Read the model definition and answer for the solid it produces. Units are mm, in the model's axes. Face numbers are marked on the shaded views. A direction names the side the tool comes from. Coordinates: 2 decimals unless noted, no trailing zeros. Order: outer loops, then holes, each group sorted by start corner. A loop starts at its lowest first (then second) coordinate and runs counter-clockwise, first axis right, second up. Notation, with made-up numbers: M 88.5,-19 L 113.5,-19 A11 ccw 113.5,-6 Z; hole C 19,77.25 d6. An arc over 180 degrees is marked long. One line per question, with ' | ' between items. Start each with the question number.
1) A tool of negligible diameter and unlimited length cuts with its end or side. For the marked faces 4, 5, 6 and 7, from which of +Z, -Z, +X, -X, +Y, -Y can it reach the whole face along a straight path? Write none if from no direction.
2) Find section A-A, the plane z = 13.2. Write down the section's boundary in (x, y).
3) Given P1, Ø4, axis at x = -12, z = 6, coming from the -Y side; P2, Ø2, axis at x = 2.5, z = -4.5, coming from the +Y side; P3, Ø2.5, axis at x = -8.5, y = 8.5, coming from the -Z side, each flat-ended and moving along its own axis, determine where each tip first touches the part or whether it passes through.
4) Find section C-C, the plane x = -9. Write down the section's boundary in (y, z).
5) Find section D-D, the plane y = -13. Write down the section's boundary in (x, z), plus the area to 3 significant figures.
6) Find section B-B, the plane y = 9. Write down the section's boundary in (x, z), plus the area to 3 significant figures.
7) The mould has two halves that part along Y. Classify the marked faces 1, 2 and 3: +Y half, -Y half, draft (parallel to the pull), parting line (faces both ways), or undercut.
8) Consider probe 1 along Y at (x, z) = (9, 1); probe 2 along Y at (x, z) = (9, -0.7); probe 3 along Z at (x, y) = (-12, -11.5). Determine where each line is inside the solid, lowest interval first.
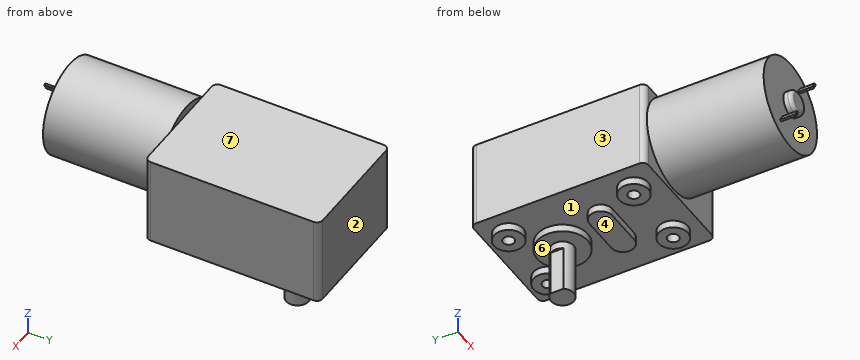
from build123d import *

# Parameters (mm, degrees)
SKETCH1_W           = 32
SKETCH1_H           = 46
BOSS_EXTRUDE1_DEPTH = 23.2
SKETCH2_R           = 3.85
SKETCH2_R_2         = 6.65
BOSS_EXTRUDE2_DEPTH = 2
SKETCH3_R           = 1.5
CUT_EXTRUDE1_DEPTH  = 4
SKETCH4_R           = 3
BOSS_EXTRUDE3_DEPTH = 14
CUT_EXTRUDE2_START  = -12
CUT_EXTRUDE2_DEPTH  = 12
FILLET1_R           = 1.5
SKETCH6_R           = 12.2
BOSS_EXTRUDE4_DEPTH = 30.8
SKETCH7_R           = 3.2
BOSS_EXTRUDE5_DEPTH = 2.2
FILLET2_R           = 1
BOSS_EXTRUDE6_DEPTH = 4


with BuildPart() as part:
    # Sketch1 → Boss-Extrude1 (new body)
    with BuildSketch(Plane.XY):
        with Locations((0, -8)):
            Rectangle(SKETCH1_W, SKETCH1_H)
    extrude(amount=BOSS_EXTRUDE1_DEPTH)

    # Sketch2 → Boss-Extrude2 (add)
    with BuildSketch(Plane(origin=(0, 0, 0), x_dir=(-1, 0, 0), z_dir=(0, 0, -1))):
        with Locations(Location((-9, 9, 0), (0, 0, 180))):
            Circle(SKETCH2_R)
        with Locations(Location((9, 9, 0), (0, 0, 180))):
            Circle(SKETCH2_R)
        with Locations(Location((-9, -24, 0), (0, 0, 180))):
            Circle(SKETCH2_R)
        with Locations(Location((9, -24, 0), (0, 0, 180))):
            Circle(SKETCH2_R)
        with Locations(Location((0, 0, 0), (0, 0, 180))):
            Circle(SKETCH2_R_2)
        with BuildLine():
            Line((-5, -10), (5, -10))
            ThreePointArc((5, -10), (8, -13), (5, -16))
            Line((5, -16), (-5, -16))
            ThreePointArc((-5, -16), (-8, -13), (-5, -10))
        make_face()
    extrude(amount=BOSS_EXTRUDE2_DEPTH)

    # Sketch3 → Cut-Extrude1 (cut)
    with BuildSketch(Plane(origin=(0, 0, -2), x_dir=(-1, 0, 0), z_dir=(0, 0, -1))):
        with Locations((9, 9)):
            Circle(SKETCH3_R)
        with Locations((-9, 9)):
            Circle(SKETCH3_R)
        with Locations((-9, -24)):
            Circle(SKETCH3_R)
        with Locations((9, -24)):
            Circle(SKETCH3_R)
    extrude(amount=-CUT_EXTRUDE1_DEPTH, mode=Mode.SUBTRACT)

    # Sketch4 → Boss-Extrude3 (add)
    with BuildSketch(Plane(origin=(0, 0, -2), x_dir=(-1, 0, 0), z_dir=(0, 0, -1))):
        Circle(SKETCH4_R)
    extrude(amount=BOSS_EXTRUDE3_DEPTH)

    # Sketch5 → Cut-Extrude2 (cut)
    with BuildSketch(Plane(origin=(0, 0, -16), x_dir=(-1, 0, 0), z_dir=(0, 0, -1)).offset(CUT_EXTRUDE2_START)):
        with BuildLine():
            Line((2.5, 1.658312395), (2.5, -1.658312395))
            ThreePointArc((2.5, -1.658312395), (2.872281323, -0.866025404), (3, 0))
            ThreePointArc((3, 0), (2.872281323, 0.866025404), (2.5, 1.658312395))
        make_face()
    extrude(amount=CUT_EXTRUDE2_DEPTH, mode=Mode.SUBTRACT)

    # Fillet1
    fillet1_edges = [part.edges().sort_by_distance(p)[0] for p in [
        (-16, 15, 11.6),
        (16, 15, 11.6),
        (16, -31, 11.6),
        (-16, -31, 11.6),
    ]]
    fillet(fillet1_edges, radius=FILLET1_R)

    # Sketch6 → Boss-Extrude4 (add)
    with BuildSketch(Plane.XZ.offset(31)):
        with Locations(Location((-3, 13.2, 0), (0, 0, 124.94801372))):
            Circle(SKETCH6_R)
    extrude(amount=BOSS_EXTRUDE4_DEPTH)

    # Sketch7 → Boss-Extrude5 (add)
    with BuildSketch(Plane.XZ.offset(61.8)):
        with Locations(Location((-3, 13.2, 0), (0, 0, 270))):
            Circle(SKETCH7_R)
    extrude(amount=BOSS_EXTRUDE5_DEPTH)

    # Fillet2
    fillet2_edges = [part.edges().sort_by_distance(p)[0] for p in [
        (-3, -64, 16.4),
    ]]
    fillet(fillet2_edges, radius=FILLET2_R)

    # Sketch8 → Boss-Extrude6 (add)
    with BuildSketch(Plane.XZ.offset(61.8)):
        with BuildLine():
            Line((1.267616567, 21.091728722), (0.299370731, 19.414677739))
            ThreePointArc((0.299370731, 19.414677739), (0.5, 19.262177826), (0.732383433, 19.164677739))
            Line((0.732383433, 19.164677739), (1.700629269, 20.841728722))
            ThreePointArc((1.700629269, 20.841728722), (1.5, 20.994228634), (1.267616567, 21.091728722))
        make_face()
        with BuildLine():
            Line((-6.299370731, 6.985322261), (-7.267616567, 5.308271278))
            ThreePointArc((-7.267616567, 5.308271278), (-7.5, 5.405771366), (-7.700629269, 5.558271278))
            Line((-7.700629269, 5.558271278), (-6.732383433, 7.235322261))
            ThreePointArc((-6.732383433, 7.235322261), (-6.5, 7.137822174), (-6.299370731, 6.985322261))
        make_face()
    extrude(amount=BOSS_EXTRUDE6_DEPTH)


solid = part.part
Report:
1) face 4: -Z, +X, -X, -Y | face 5: -Y | face 6: -Z | face 7: +Z, +X, -X, +Y
2) outline: M -16,-29.5 A1.5 ccw -14.5,-31 L -15.2,-31 L -15.2,-61.8 L -6.2,-61.8 L -6.2,-63 A1 ccw -5.2,-64 L -0.8,-64 A1 ccw 0.2,-63 L 0.2,-61.8 L 9.2,-61.8 L 9.2,-31 L 14.5,-31 A1.5 ccw 16,-29.5 L 16,13.5 A1.5 ccw 14.5,15 L -14.5,15 A1.5 ccw -16,13.5 Z
3) P1: stops at y = -61.8 | P2: stops at y = 2.6 | P3: stops at z = -2
4) outline: M -61.8,2.58 L -31,2.58 L -31,0 L -27.85,0 L -27.85,-2 L -25.5,-2 L -25.5,2 L -22.5,2 L -22.5,-2 L -20.15,-2 L -20.15,0 L 5.15,0 L 5.15,-2 L 7.5,-2 L 7.5,2 L 10.5,2 L 10.5,-2 L 12.85,-2 L 12.85,0 L 15,0 L 15,23.2 L -31,23.2 L -31,23.82 L -61.8,23.82 Z
5) outline: M -16,0 L -8,0 L -8,-2 L 8,-2 L 8,0 L 16,0 L 16,23.2 L -16,23.2 Z | area: 774 mm^2
6) outline: M -16,0 L -12.85,0 L -12.85,-2 L -10.5,-2 L -10.5,2 L -7.5,2 L -7.5,-2 L -5.15,-2 L -5.15,0 L 5.15,0 L 5.15,-2 L 7.5,-2 L 7.5,2 L 10.5,2 L 10.5,-2 L 12.85,-2 L 12.85,0 L 16,0 L 16,23.2 L -16,23.2 Z | area: 749 mm^2
7) face 1: undercut | face 2: +Y half | face 3: draft
8) probe 1: y = -31 to -25.5, -22.5 to 7.5, 10.5 to 15 | probe 2: y = -27.85 to -25.5, -22.5 to -20.15, 5.15 to 7.5, 10.5 to 12.85 | probe 3: z = 0 to 23.2
